from build123d import *

# Parameters (mm, degrees)
BOSS_EXTRUDE1_DEPTH = 15
BOSS_EXTRUDE2_DEPTH = 245
BOSS_EXTRUDE3_DEPTH = 245
BOSS_EXTRUDE4_DEPTH = 245
CUT_EXTRUDE1_DEPTH  = 245
CHAMFER1_SIZE       = 12


with BuildPart() as part:
    # Sketch1 → Boss-Extrude1 (new body)
    with BuildSketch(Plane.XY):
        with BuildLine():
            Line((15, 15), (260, 15))
            ThreePointArc((260, 15), (86.758838609, 86.758838609), (15, 260))
            Line((15, 260), (15, 15))
        make_face()
    extrude(amount=BOSS_EXTRUDE1_DEPTH)

    # Sketch2 → Boss-Extrude2 (add)
    with BuildSketch(Plane.XZ.offset(-15)):
        Polygon((15, 0), (0, 15), (15, 15), align=None)
    extrude(amount=-BOSS_EXTRUDE2_DEPTH)

    # Sketch3 → Boss-Extrude3 (add)
    with BuildSketch(Plane(origin=(15, 0, 0), x_dir=(0, 0, -1), z_dir=(1, 0, 0))):
        Polygon((0, 15), (-15, 0), (-15, 15), align=None)
    extrude(amount=BOSS_EXTRUDE3_DEPTH)

    # Sketch4 → Boss-Extrude4 (add)
    with BuildSketch(Plane.ZY.offset(-15)):
        Polygon((15, 15), (0, 15), (15, 0), align=None)
    extrude(amount=BOSS_EXTRUDE4_DEPTH)

    # Sketch5 → Cut-Extrude1 (cut)
    with BuildSketch(Plane(origin=(0, 15, 0), x_dir=(1, 0, 0), z_dir=(0, 1, 0))):
        Polygon((0, -15), (15, 0), (-230, 0), (-230, -15), align=None)
    extrude(amount=-CUT_EXTRUDE1_DEPTH, mode=Mode.SUBTRACT)

    # Chamfer1
    chamfer1_edges = [part.edges().sort_by_distance(p)[0] for p in [
        (86.758838609, 86.758838609, 15),
    ]]
    chamfer(chamfer1_edges, length=CHAMFER1_SIZE)


solid = part.part
Can you work these out from the model? Positions are in its coordinate system, mm. Round coordinates to 2 decimals unless told otherwise and drop trailing zeros. Loops run counter-clockwise (first coordinate to the right, second up) from the corner with the lowest first, then second, coordinate; pieces in that order, holes last. Notation, with made-up numbers: (-14.75, 46) - (-3.75, 46) arc R29 ccw to (-3.75, 70) - close; hole circle Ø4 at (61, 24). An arc over 180 degrees is marked (long way). Answer in a Markdown table with one row per item. Add a question column.
Q1. We'd pull the mould along Z, two halves only. Please class faces 1 (the flat face through (8, 260, 9)), 2 (the flat face through (54, 62, 15)), 3 (the flat face through (8, 128, 7)): pulls with the +Z half, pulls with the -Z half, needs draft (parallel to the pull), parting line crosses it, or undercut.
Q2. I need wall thicknesses on L1, parallel to X at y = 211.5, z = 2.5; L2, parallel to Y at x = 121, z = 4.5; L3, parallel to X at y = 246.5, z = 10.5. Which ranges of each line are inside material? Lowest first, please.
Q3. For pin 1 Ø6 at (y, z) = (76, 5) entering from -X; pin 2 Ø8 at (y, z) = (104.5, 9) entering from -X; pin 3 Ø1.5 at (x, z) = (212.5, 1.5) entering from -Y, each with a flat end and sliding along its axis, tell me the tip position at first contact or that it passes through.
Q4. I want a section at A-A on z = 11.5. List the corners of the cut face in (x, y) for me, and give its area (3 significant figures).
A:
| question | item | result |
|---|---|---|
| 1 | face 1 | needs draft |
| 1 | face 2 | pulls with the +Z half |
| 1 | face 3 | pulls with the -Z half |
| 2 | L1 | 12.5 to 19.85 |
| 2 | L2 | 10.5 to 56.43 |
| 2 | L3 | 4.5 to 7.86 |
| 3 | pin 1 | x = 7 |
| 3 | pin 2 | x = 2 |
| 3 | pin 3 | y = 12.75 |
| 4 | outline | (3.5, 3.5) - (260, 3.5) - (260, 6.5) arc R253.5 cw to (6.5, 260) - (3.5, 260) - close |
| 4 | area | 15,300 mm^2 |
